Here's how the part is built. I have some questions about the finished solid (model axes, mm). A direction names the side the tool comes from. Give positions to 0.01 mm unless a question says otherwise; leave off trailing zeros. Loops run counter-clockwise (first coordinate to the right, second up) from the corner with the lowest first, then second, coordinate; pieces in that order, holes last.
Q1. Suppose I cut it at B-B (x = 92.5). List the corners of the cut face in (y, z) for me.
Q2. I'm going to push flat-ended pins straight in: P1, Ø10, axis at x = 100, z = 82.5, coming from the +Y side; P2, Ø1.5, axis at x = 147, z = 80, coming from the -Y side; P3, Ø6, axis at x = 109, y = 120, coming from the -Z side. Where does each tip first touch, or does it pass through?
Q3. Thinking about a two-plate mould opening in X: for faces 3 (the face through (102.96, -12.39, 50.3)), 4 (the face through (92, 0, 54)), 5 (the face through (49.85, 57, 54)), 6 (the face through (159.024, 57, 54)), which applies, pulls with the +X half, pulls with the -X half, needs draft (parallel to the pull), parting line crosses it, or undercut?
Q4. For faces 1 (the face through (104, 59, 110)), 2 (the face through (102.96, 130.35, 50.3)), which set-ups out of +Z, -Z, +X, -X, +Y, -Y let a thin tool reach every point of the face, with its end or its side?
Q5. Suppose I cut it at D-D (z = 79). List the corners of the cut face in (x, y) for me.
Q6. Suppose I cut it at A-A (z = 55). List the corners of the cut face in (x, y) for me, and give its area (3 significant figures).
Q7. Suppose I cut it at C-C (y = -7). List the corners of the cut face in (x, z) for me, and give its area (3 significant figures).
Q8. I need wall thicknesses on probe 1 along Y at (x, z) = (104, 27.5). Which ranges of the line are inside material? Lowest first, please.
```python
from build123d import *

# Parameters (mm, degrees)
SKETCH_1_W           = 109.173065233
SKETCH_1_H           = 115.560150299
EXTRUDE_1_DEPTH      = 110
EXTRUDE_2_DEPTH      = 30
EXTRUDE_2_DEPTH_BACK = 140
SKETCH_2_R           = 4.92730672


with BuildPart() as part:
    # 草图1 → 凸台-拉伸1 (new body)
    with BuildSketch(Plane.XY):
        with Locations((104.436974975, 57.78007515)):
            Rectangle(SKETCH_1_W, SKETCH_1_H)
    extrude(amount=EXTRUDE_1_DEPTH)

    # 草图2 → 凸台-拉伸2 (add, two sides: drawn at the far end of the back side and taken through both)
    with BuildSketch(Plane(origin=(0, 115.560150299, 0), x_dir=(1, 0, 0), z_dir=(0, 1, 0)).offset(-EXTRUDE_2_DEPTH_BACK)):
        with Locations(Location((104.436974975, -55, 0), (0, 0, 90))):
            Circle(SKETCH_2_R)
    extrude(amount=EXTRUDE_2_DEPTH + EXTRUDE_2_DEPTH_BACK)


solid = part.part
```
Solutions:
1. outline: (0, 0) - (115.56, 0) - (115.56, 110) - (0, 110) - close
2. P1: stops at y = 115.56
2. P2: stops at y = 0
2. P3: stops at z = 50.33
3. face 3: parting line crosses it
3. face 4: needs draft
3. face 5: pulls with the -X half
3. face 6: pulls with the +X half
4. face 1: +Z, +X, -X, +Y, -Y
4. face 2: +Y
5. outline: (49.85, 0) - (159.02, 0) - (159.02, 115.56) - (49.85, 115.56) - close
6. outline: (49.85, 0) - (99.51, 0) - (99.51, -24.44) - (109.36, -24.44) - (109.36, 0) - (159.02, 0) - (159.02, 115.56) - (109.36, 115.56) - (109.36, 145.56) - (99.51, 145.56) - (99.51, 115.56) - (49.85, 115.56) - close
6. area: 13,200 mm2
7. outline: circle Ø9.85 at (104.44, 55)
7. area: 76.3 mm2
8. probe 1: y = 0 to 115.56
